```python
from build123d import *

# Parameters (mm, degrees)
F0_W     = 500
F0_H     = 170
F1_DEPTH = 3
F3_DEPTH = 500
F5_D     = 3
F5_DEPTH = 25


with BuildPart() as f1:
    # F0 (on Front) → F1 (new body)
    with BuildSketch(Plane.XZ):
        with Locations((61.018479, 12.994566)):
            Rectangle(F0_W, F0_H)
    extrude(amount=F1_DEPTH)

    # F2 (on face) → F3 (join, through all)
    with BuildSketch(Plane.YZ.offset(311.018479)):
        Polygon((0, 97.994566), (0, 87.994566), (10, 87.994566), (10, 97.994566), (9, 96.994566), (9, 88.994566), (1, 88.994566), (1, 96.994566), align=None)
    extrude(amount=-F3_DEPTH)

    # F5
    with Locations(Plane.XZ.offset(3)):
        with Locations((61.018479, -2.005434), (81.018479, 23.994566), (121.018479, 23.994566), (161.018479, -2.005434), (209.018479, 54.994566), (239.018479, 54.994566)):
            Hole(F5_D / 2, depth=F5_DEPTH)


solid = f1.part
```
Geometry: final body of the model. Coordinates: model frame, mm. A direction names the side the tool comes from. Give positions to 0.01 mm unless a question says otherwise; leave off trailing zeros. Write each loop counter-clockwise with the first axis right and the second up, starting at its lowest first coordinate (ties: lowest second). Pieces come first, ordered by that corner, then holes.
1. Section query B-B, the plane z = -29. Return loops of the section in (x, y), then the cut area to 3 significant figures.
2. Reachability of faces 1 (the flat face through (65, 5, 87.995)), 2 (the flat face through (58, -3, 14)), 3 (the flat face through (65, 5, 88.995)) from +Z, -Z, +X, -X, +Y, -Y: full face, straight path, thin tool, end or side. Return the list, or none.
3. Line query: probe 1 along Z at (x, y) = (215, 7.75); probe 2 along Y at (x, z) = (-104, 87); probe 3 along Z at (x, y) = (89.5, 0.25). Output: solid intervals per line, ascending.
4. Section query C-C, the plane y = 3.5. Return loops of the section in (x, z), then the cut area to 3 significant figures.
5. Section query A-A, the plane x = -88. Return loops of the section in (y, z).
6. Draft query along Y for faces 4 (the flat face through (65, 10, 93)), 5 (the flat face through (311.018, -2, 20)), 6 (the flat face through (65, 1, 93)). Return one class per face: released by +Y, released by -Y, zero draft, split by the parting line, or undercut.
7. Pin query (flat end, axial travel): P1, Ø2, axis at x = 245.5, y = 3.5, coming from the -Z side; P2, Ø4, axis at x = 121.02, z = 23.99, coming from the -Y side; P3, Ø5, axis at x = 61.02, z = -2.01, coming from the +Y side; P4, Ø1.5, axis at x = 147, y = 4, coming from the +Z side. Return the tip coordinate at first contact, or that it passes through.
Computed:
1. outline: (-188.98, -3) - (311.02, -3) - (311.02, 0) - (-188.98, 0) - close
1. area: 1,500 mm2
2. face 1: -Z, +X, -X, +Y
2. face 2: +Z, -Z, +X, -X, -Y
2. face 3: +Z, +X, -X
3. probe 1: z = 87.99 to 88.99
3. probe 2: y = -3 to 0
3. probe 3: z = 87.99 to 97.74
4. outline: (-188.98, 87.99) - (311.02, 87.99) - (311.02, 88.99) - (-188.98, 88.99) - close
4. area: 500 mm2
5. outline: (-3, -72.01) - (0, -72.01) - (0, 87.99) - (10, 87.99) - (10, 97.99) - (9, 96.99) - (9, 88.99) - (1, 88.99) - (1, 96.99) - (0, 97.99) - (-3, 97.99) - close
6. face 4: released by +Y
6. face 5: zero draft
6. face 6: undercut
7. P1: stops at z = 87.99
7. P2: stops at y = -3
7. P3: stops at y = 0
7. P4: stops at z = 88.99
